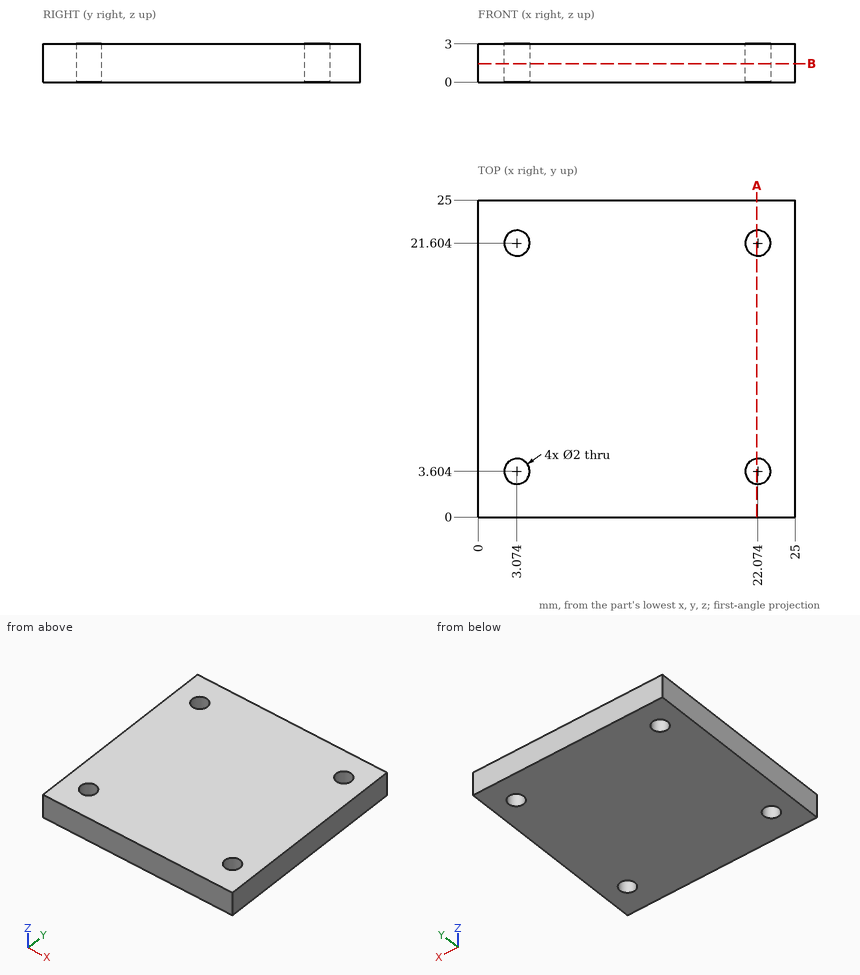
Check sheet for the drawn part. Datum: minimum x, y, z corner. Units: mm. Round coordinates to 2 decimals unless told otherwise and drop trailing zeros. Loops run counter-clockwise (first coordinate to the right, second up) from the corner with the lowest first, then second, coordinate; pieces in that order, holes last. Notation, with made-up numbers: (87, 29) -> (105, 29) arc R10 cw to (105, 41) -> close; hole circle Ø5 at (-31, 29.25). An arc over 180 degrees is marked (long way). Put each result on its own line as item: value. Start each with the question number.
1. Section check B-B (z = 1.45). Enter the section's corners in (x, y).
2. Section check A-A (x = 22). Enter the section's corners in (y, z).
3. Scan lines: probe 1 along X at (y, z) = (3.5, 1.25); probe 2 along X at (y, z) = (22, 2.7) (1 decimal); probe 3 along Y at (x, z) = (2.25, 0.6) (1 decimal). Record each from-to range of solid material in increasing order.
Findings:
1. outline: (0, 0) -> (25, 0) -> (25, 25) -> (0, 25) -> close; hole circle Ø2 at (3.07, 3.6); hole circle Ø2 at (3.07, 21.6); hole circle Ø2 at (22.07, 3.6); hole circle Ø2 at (22.07, 21.6)
2. outline: (0, 0) -> (2.61, 0) -> (2.61, 3) -> (0, 3) -> close; (4.6, 0) -> (20.61, 0) -> (20.61, 3) -> (4.6, 3) -> close; (22.6, 0) -> (25, 0) -> (25, 3) -> (22.6, 3) -> close
3. probe 1: x = 0 to 2.08, 4.07 to 21.08, 23.07 to 25
3. probe 2: x = 0 to 2.2, 4 to 21.2, 23 to 25
3. probe 3: y = 0 to 3, 4.2 to 21, 22.2 to 25
